Design review of the part built by this model. Coordinates are the model's own, in mm. A direction names the side the tool comes from. Give positions to 0.01 mm unless a question says otherwise; leave off trailing zeros. Loops run counter-clockwise (first coordinate to the right, second up) from the corner with the lowest first, then second, coordinate; pieces in that order, holes last. Notation, with made-up numbers: M 0.25,56 L 51.25,56 A10 ccw 51.25,61 Z; hole C 75.25,56 d1. An arc over 180 degrees is marked long. Answer as CSV lines item,"result".
```python
from build123d import *

# Parameters (mm, degrees)
SKETCH1_R           = 1.5
SKETCH1_W           = 18.658985537
SKETCH1_H           = 31.487038094
BOSS_EXTRUDE1_DEPTH = 5


with BuildPart() as part:
    # Sketch1 → Boss-Extrude1 (new body)
    with BuildSketch(Plane(origin=(0, 0, 0), x_dir=(1, 0, 0), z_dir=(0, 1, 0))):
        Polygon((-124.555160142, -60.782918149), (155.444839858, -60.782918149), (155.444839858, 9.217081851), (-32.555160142, 9.217081851), (-32.555160142, 89.217081851), (-124.555160142, 89.217081851), align=None)
        with Locations(Location((-96.88048066, -44.579371447, 0), (0, 0, 270))):
            Circle(SKETCH1_R, mode=Mode.SUBTRACT)
        with Locations(Location((-57.609979708, -55.025558837, 0), (0, 0, 270))):
            Circle(SKETCH1_R, mode=Mode.SUBTRACT)
        with Locations(Location((-49.124698334, -46.540277462, 0), (0, 0, 270))):
            Circle(SKETCH1_R, mode=Mode.SUBTRACT)
        with Locations(Location((-96.88048066, -4.623906574, 0), (0, 0, 270))):
            Circle(SKETCH1_R, mode=Mode.SUBTRACT)
        with Locations(Location((82.11951934, -44.623906574, 0), (0, 0, 270))):
            Circle(SKETCH1_R, mode=Mode.SUBTRACT)
        with Locations(Location((109.860128873, -55.261198979, 0), (0, 0, 270))):
            Circle(SKETCH1_R, mode=Mode.SUBTRACT)
        with Locations(Location((114.620218271, -46.782918149, 0), (0, 0, 270))):
            Circle(SKETCH1_R, mode=Mode.SUBTRACT)
        with Locations(Location((118.345410248, -46.775917605, 0), (0, 0, 270))):
            Circle(SKETCH1_R, mode=Mode.SUBTRACT)
        with Locations(Location((141.300092758, -46.782918149, 0), (0, 0, 270))):
            Circle(SKETCH1_R, mode=Mode.SUBTRACT)
        with Locations((129.159877134, -24.440324762)):
            Rectangle(SKETCH1_W, SKETCH1_H, mode=Mode.SUBTRACT)
        with Locations(Location((82.11951934, -4.623906574, 0), (0, 0, 270))):
            Circle(SKETCH1_R, mode=Mode.SUBTRACT)
        with Locations(Location((114.620218271, -1.782918149, 0), (0, 0, 270))):
            Circle(SKETCH1_R, mode=Mode.SUBTRACT)
        with Locations(Location((141.300092758, -1.782918149, 0), (0, 0, 270))):
            Circle(SKETCH1_R, mode=Mode.SUBTRACT)
        with Locations(Location((-37.752255096, 83.459722538, 0), (0, 0, 270))):
            Circle(SKETCH1_R, mode=Mode.SUBTRACT)
        with Locations(Location((-109.616514697, 27.990725731, 0), (0, 0, 270))):
            Circle(SKETCH1_R, mode=Mode.SUBTRACT)
        with Locations(Location((-118.326917326, 29.495275711, 0), (0, 0, 270))):
            Circle(SKETCH1_R, mode=Mode.SUBTRACT)
        with Locations(Location((-109.616514697, 49.990725731, 0), (0, 0, 270))):
            Circle(SKETCH1_R, mode=Mode.SUBTRACT)
        with Locations(Location((-49.316514697, 27.990725731, 0), (0, 0, 270))):
            Circle(SKETCH1_R, mode=Mode.SUBTRACT)
        with Locations(Location((-38.326917326, 29.495275711, 0), (0, 0, 270))):
            Circle(SKETCH1_R, mode=Mode.SUBTRACT)
        with Locations(Location((-49.316514697, 49.990725731, 0), (0, 0, 270))):
            Circle(SKETCH1_R, mode=Mode.SUBTRACT)
        with Locations(Location((-118.326917326, 69.495275711, 0), (0, 0, 270))):
            Circle(SKETCH1_R, mode=Mode.SUBTRACT)
        with Locations(Location((-38.326917326, 69.495275711, 0), (0, 0, 270))):
            Circle(SKETCH1_R, mode=Mode.SUBTRACT)
        with Locations(Location((-46.23753647, 74.974441163, 0), (0, 0, 270))):
            Circle(SKETCH1_R, mode=Mode.SUBTRACT)
    extrude(amount=BOSS_EXTRUDE1_DEPTH)


solid = part.part
```
1. We need section B-B, the plane y = 3.85. Count the separate pieces of the cut face and the enclosed holes in it, plus the area to 3 significant figures.
Answer block:
separate pieces,"1"
enclosed holes,"23"
area,"26,200 mm²"
2. To check wall thickness, follow L1, parallel to X at y = 1.45, z = 5; L2, parallel to X at y = 2.4, z = -68.5; L3, parallel to Z at x = 121.5, y = 3.15. State the ranges of each line that lie inside material, in increasing order. Write a range as [from, to].
Answer block:
L1,"[-124.56, -98.33], [-95.43, 80.67], [83.57, 155.44]"
L2,"[-124.56, -119.45], [-117.2, -39.45], [-37.2, -32.56]"
L3,"[-9.22, 8.7], [40.18, 60.78]"
3. For P1, Ø4, axis at x = 109.86, z = 55.26, coming from the +Y side; P2, Ø1.5, axis at x = 93.5, y = 2.5, coming from the -Z side, all flat-tipped, find the tip position at first contact; note any pin that passes through.
Answer block:
P1,"y = 5"
P2,"z = -9.22"
4. The part is to be moulded in two halves that separate along Z. For faces 1 (the flat face through (155.445, 2, 26)), 2 (the flat face through (-78, 2, -89.217)), 3 (the flat face through (138.489, 2, 25)), 4 (the flat face through (129, 2, 40.184)), say which applies: pulls with the +Z half, pulls with the -Z half, needs draft (parallel to the pull), parting line crosses it, or undercut.
Answer block:
face 1,"needs draft"
face 2,"pulls with the -Z half"
face 3,"undercut"
face 4,"undercut"
5. For faces 5 (the flat face through (119.83, 2, 25)), 6 (the flat face through (13, 2, 60.783)), 7 (the flat face through (-32.555, 2, -49)), list the 3-axis set-ups (+Z, -Z, +X, -X, +Y, -Y) from which the entire face can be reached by the end or side of a thin tool; tool diameter is ignored.
Answer block:
face 5,"+Y, -Y"
face 6,"+Z, +X, -X, +Y, -Y"
face 7,"-Z, +X, +Y, -Y"
6. We need section A-A, the plane z = 23. Write out the cut boundary in (x, y), plus the area to 3 significant figures.
Answer block:
outline,"M -124.56,0 L 119.83,0 L 119.83,5 L -124.56,5 Z; M 138.49,0 L 155.44,0 L 155.44,5 L 138.49,5 Z"
area,"1,310 mm²"
7. We need section C-C, the plane x = -6. Write out the cut boundary in (y, z).
Answer block:
outline,"M 0,-9.22 L 5,-9.22 L 5,60.78 L 0,60.78 Z"
